Design review of the part built by this model. Coordinates are the model's own, in mm. Face numbers are marked on the shaded views. A direction names the side the tool comes from. Coordinates: 2 decimals unless noted, no trailing zeros. Loops run counter-clockwise (first coordinate to the right, second up) from the corner with the lowest first, then second, coordinate; pieces in that order, holes last. Notation, with made-up numbers: M -11,87.5 L 2,87.5 A9 cw 2,104.5 Z; hole C 46.25,2 d4. An arc over 180 degrees is marked long. One line per item, written item: value.
```python
from build123d import *

# Parameters (mm, degrees)
F1_DEPTH = 22.86
F2_W     = 23.88052
F2_H     = 21.403259
F3_DEPTH = 20.32
F5_DEPTH = 20.32


with BuildPart() as f1:
    # F0 (on Top) → F1 (new body)
    with BuildSketch(Plane.XY):
        Polygon((-45.509029, 47.247883), (-45.808434, -41.675467), (53.594097, -41.675467), (53.594097, 47.247883), align=None)
    extrude(amount=F1_DEPTH)

    # F2 (on face) → F3 (join)
    with BuildSketch(Plane.XY.offset(22.86)):
        with Locations((41.653837, 36.546253)):
            Rectangle(F2_W, F2_H)
    extrude(amount=F3_DEPTH)

    # F4 (on face) → F5 (join)
    with BuildSketch(Plane.XY.offset(22.86)):
        Polygon((-25.999382, 27.392207), (-25.999382, 47.247883), (-45.509029, 47.247883), (-45.575883, 27.392207), align=None)
    extrude(amount=F5_DEPTH)


solid = f1.part
```
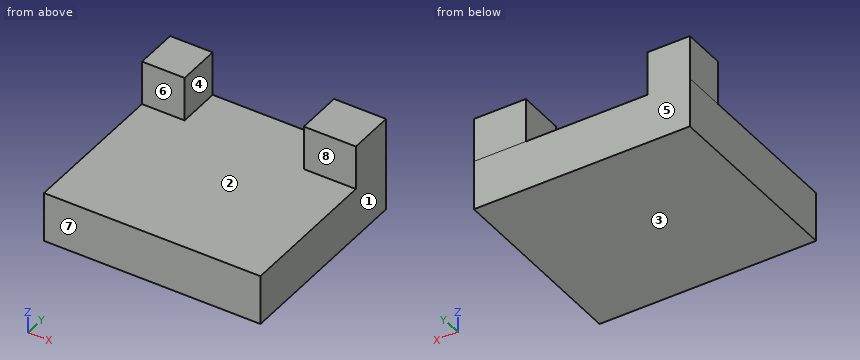
(1) Insertion check: pin 1 (1.5 mm diameter, centred on y = 3.5, z = 15.5, fed in from -X); pin 2 (4 mm diameter, centred on x = 32.5, z = 29, fed in from -Y); pin 3 (1 mm diameter, centred on x = -34.5, y = 30.5, fed in from -Z); pin 4 (6 mm diameter, centred on y = 38, z = 29.5, fed in from -X). Each pin has a flat end and moves straight along its axis. Give the tip position at first contact, or say it passes through.
Reply:
pin 1: stops at x = -45.66
pin 2: stops at y = 25.84
pin 3: stops at z = 0
pin 4: stops at x = -45.55
(2) To check wall thickness, follow line 1 along X through (y, z) = (42, 37); line 2 along Z through (x, y) = (23, -13.5); line 3 along X through (y, z) = (30, 14). State the ranges of each line that lie inside material, in increasing order. Write a range as [from, to].
Reply:
line 1: x = [-45.53, -26], [29.71, 53.59]
line 2: z = [0, 22.86]
line 3: x = [-45.57, 53.59]
(3) Mouldability with a two-part tool opening along X and no side actions: class the marked faces 1, 2 and 3 as released by +X, released by -X, zero draft, split by the parting line, or undercut.
Reply:
face 1: released by +X
face 2: undercut
face 3: zero draft
(4) We need section D-D on x = 21.5. State the section outline as (y, z) points.
Reply:
outline: M -41.68,0 L 47.25,0 L 47.25,22.86 L -41.68,22.86 Z
(5) We need section B-B on x = -33. State the section outline as (y, z) points, then the cut area to 3 significant figures.
Reply:
outline: M -41.68,0 L 47.25,0 L 47.25,43.18 L 27.39,43.18 L 27.39,22.86 L -41.68,22.86 Z
area: 2,440 mm2
(6) Tool access review of the marked faces 4, 5, 6, 7 and 8: name each direction out of +Z, -Z, +X, -X, +Y, -Y from which nothing blocks a thin tool from reaching the whole face with its end or side.
Reply:
face 4: +Z, +Y, -Y
face 5: +Z, -Z, +X, -X, +Y
face 6: +Z, -X, -Y
face 7: +Z, -Z, +X, -X, -Y
face 8: +Z, +X, -X, -Y
(7) We need section C-C on y = 38. State the section outline as (x, z) points.
Reply:
outline: M -45.54,0 L 53.59,0 L 53.59,43.18 L 29.71,43.18 L 29.71,22.86 L -26,22.86 L -26,43.18 L -45.54,43.18 Z
(8) We need section A-A on z = 29. State the section outline as (x, y) points, then the cut area to 3 significant figures.
Reply:
outline: M -45.58,27.39 L -26,27.39 L -26,47.25 L -45.51,47.25 Z; M 29.71,25.84 L 53.59,25.84 L 53.59,47.25 L 29.71,47.25 Z
area: 899 mm2
